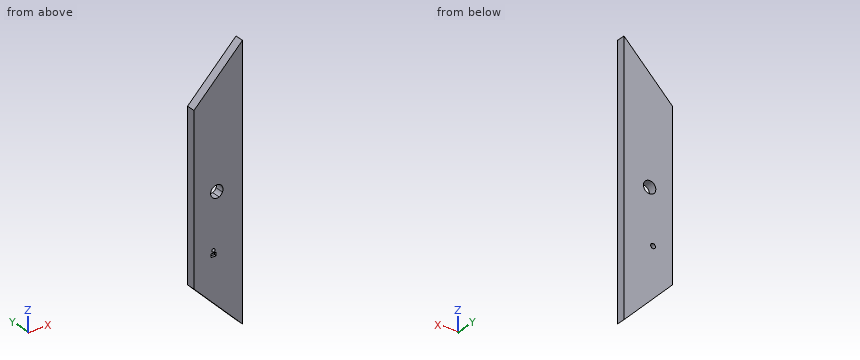
Autodesk Inventor part; units mm, degrees
ref_plane "YZ Plane" through (0, 0, 0) normal (1, 0, 0) x (0, 1, 0)
ref_plane "XZ Plane" through (0, 0, 0) normal (0, 1, 0) x (-1, 0, 0)
ref_plane "XY Plane" through (0, 0, 0) normal (0, 0, 1) x (1, 0, 0)
sketch "Sketch1" plane through (0, 0, 0) normal (0, 1, 0) x (-1, 0, 0)
  line L0 (0, 0) -> (0, -340)
  line L1 (0, 0) -> (-100, 0)
  line L2 (-100, 0) -> (-100, 100)
  line L3 (-100, 100) -> (0, 0)
  line L4 (0, -340) -> (-100, -340)
  line L5 (-100, -340) -> (-100, -440)
  line L6 (-100, -440) -> (0, -340)
  line L7 (-100, -340) -> (-100, 0)
  dimension "d0" = 340
  dimension "d1" = 100
  dimension "d2" = 100
  dimension "d3" = 100
  dimension "d4" = 100
extrude "Extrusion1" add sketch "Sketch1" along normal blind 18
sketch "Sketch2" plane through (0, 0, 0) normal (0, -1, 0) x (1, 0, 0)
  line L0 (70, -367.7995) -> (70, -407.7995)
  line L1 (25, 17.2005) -> (25, -362.7995)
  arc A0 (51.7994, -181.8328) -> (58.8525, -174.9214) centre (47.1172, -170) ccw
  circle A1 centre (47.1172, -170) radius 12.7255
  line L2 (0, -340) -> (100, -440)
  line L3 (100, 100) -> (0, 0)
  line L4 (100, -440) -> (100, 100)
  line L5 (0, 0) -> (0, -340)
  line L6 (100, 100) -> (100, -440)
  line L7 (100, -170) -> (0, -170)
  point P0 (30, 22.2005)
extrude "Extrusion2" cut sketch "Sketch2" against normal blind 20 contours A1 L7 A0 | A1 L7
sketch "Sketch4" plane through (0, 18, 0) normal (0, 1, 0) x (1, 0, 0)
  circle A0 centre (40.0978, 279.5843) radius 3.2826
  line L0 (35.3115, 284.709) -> (45.7543, 284.709)
  line L1 (45.7543, 284.709) -> (45.7543, 291.8643)
  line L2 (45.7543, 291.8643) -> (35.3115, 291.8643)
  line L3 (35.3115, 291.8643) -> (35.3115, 284.709)
  line L4 (0, 340) -> (0, 0)
  line L5 (0, 340) -> (100, 440)
  line L6 (100, -100) -> (100, 440)
  line L7 (100, -100) -> (0, 0)
  dimension "d24" = 6.5652
extrude "Extrusion4" cut sketch "Sketch4" against normal blind 10 contours A0
sketch "Sketch6" plane through (0, 0, 0) normal (0, -1, 0) x (1, 0, 0)
  circle A0 centre (40.0978, -279.5843) radius 3.2826
  circle A1 centre (40.0978, -279.5843) radius 3.2826
  circle A2 centre (40.0978, -279.5843) radius 5
  point P0 (0, 0)
  dimension "d14" = 10
sketch "Sketch7" plane through (0, 18, 0) normal (0, 1, 0) x (1, 0, 0)
  circle A0 centre (40.0978, 279.5843) radius 3.2826
  line L0 (35.3115, 284.709) -> (45.7543, 284.709)
  line L1 (45.7543, 284.709) -> (45.7543, 291.8643)
  line L2 (45.7543, 291.8643) -> (35.3115, 291.8643)
  line L3 (35.3115, 291.8643) -> (35.3115, 284.709)
  line L4 (0, 340) -> (0, 0)
  line L5 (0, 340) -> (100, 440)
  line L6 (100, -100) -> (100, 440)
  line L7 (100, -100) -> (0, 0)
  circle A1 centre (40.0978, 279.5843) radius 5
  dimension "d19" = 10
extrude "Extrusion7" cut sketch "Sketch7" against normal blind 10 contours A0 | A1
extrude "Extrusion8" cut sketch "Sketch6" against normal blind 18 contours A0
sketch "Sketch9" plane through (0, 0, 0) normal (0, -1, 0) x (1, 0, 0)
  circle A0 centre (40.0978, -279.5843) radius 3.2826
  circle A1 centre (47.1172, -170) radius 12.7255
  line L0 (0, 0) -> (100, 100)
  line L1 (0, -340) -> (0, 0)
  line L2 (100, -440) -> (0, -340)
  line L3 (100, 100) -> (100, -440)
  line L4 (35.3092, -291.8611) -> (45.7546, -291.8611)
  line L5 (45.7546, -291.8611) -> (45.7546, -284.7095)
  line L6 (45.7546, -284.7095) -> (35.3092, -284.7095)
  line L7 (35.3092, -284.7095) -> (35.3092, -291.8611)
extrude "Extrusion9" cut sketch "Sketch9" against normal blind 5 contours L7 L6 L5 L4
properties part number "Fata_2"
Design review of the part built by this model. Coordinates are the model's own, in mm. Coordinates: 2 decimals unless noted, no trailing zeros. Loops run counter-clockwise (first coordinate to the right, second up) from the corner with the lowest first, then second, coordinate; pieces in that order, holes last. Notation, with made-up numbers: (88, 70.25) - (104, 70.25) arc R19 cw to (104, 77.25) - close; hole circle Ø6 at (-18, 62.25). An arc over 180 degrees is marked (long way). Use CSV: the item, a comma, the result in double quotes. Start each with the question number.
1. Clearance check with flat-ended pins moving along their axes: pin 1 (4 mm diameter, centred on x = 72.5, y = 13, fed in from -Z); pin 2 (5 mm diameter, centred on x = 41.5, z = -278, fed in from +Y); pin 3 (3 mm diameter, centred on x = 40, y = 14, fed in from -Z); pin 4 (4 mm diameter, centred on y = 1.5, z = -289, fed in from -X). State where each tip first meets the part, or that it passes through.
2. Add section A-A on z = -170. Give the boundary of the cut face in (x, y).
3. Add section B-B on y = 14. Give the boundary of the cut face in (x, z).
4. Add section C-C on z = 5. Give the boundary of the cut face in (x, y).
5. Add section D-D on x = 18.5. Give the boundary of the cut face in (y, z), plus the area to 3 significant figures.
6. To check wall thickness, follow probe 1 along X at (y, z) = (10.25, -170); probe 2 along Z at (x, y) = (39.5, 15); probe 3 along Z at (x, y) = (38.5, 3.5). State the ranges of each line that lie inside material, in increasing order.
Resolved:
1,pin 1,"z = -414.5"
1,pin 2,"y = 8"
1,pin 3,"z = -381.5"
1,pin 4,"x = 0"
2,outline,"(0, 0) - (34.39, 0) - (34.39, 18) - (0, 18) - close; (59.84, 0) - (100, 0) - (100, 18) - (59.84, 18) - close"
3,outline,"(0, -340) - (100, -440) - (100, 100) - (0, 0) - close; hole circle Ø10 at (40.1, -279.58); hole (51.8, -181.83) arc R12.73 ccw to (58.85, -174.92) arc R12.73 ccw (long way) to start"
4,outline,"(5, 0) - (100, 0) - (100, 18) - (5, 18) - close"
5,outline,"(0, -358.5) - (18, -358.5) - (18, 18.5) - (0, 18.5) - close"
5,area,"6,790 mm2"
6,probe 1,"0 to 34.39, 59.84 to 100"
6,probe 2,"-379.5 to -284.55, -274.62 to -180.19, -159.81 to 39.5"
6,probe 3,"-378.5 to -291.86, -284.71 to -282.45, -276.72 to -179.36, -160.64 to 38.5"
